```python
from build123d import *

# Parameters (mm, degrees)
SKICA1_R                = 2
P_IDAT_VYSUNUT_M3_DEPTH = 2


with BuildPart() as part:
    # Skica1 → Přidat vysunutím3 (new body)
    # profile 1 of 2: a face of its own
    with BuildSketch(Plane(origin=(0, 0, 0), x_dir=(1, 0, 0), z_dir=(0, 1, 0))):
        with BuildLine():
            Line((108.040914438, 105.971068272), (106.006427981, 34.226677149))
            ThreePointArc((106.006427981, 34.226677149), (110.004588085, 37.999997369), (113.994081517, 34.217515135))
            Line((113.994081517, 34.217515135), (112.040914438, 106))
            Line((112.040914438, 106), (110, 111.642221926))
            Line((110, 111.642221926), (108.040914438, 105.971068272))
        make_face()
    # profile 2 of 2: a face of its own
    with BuildSketch(Plane(origin=(0, 0, 0), x_dir=(1, 0, 0), z_dir=(0, 1, 0))):
        with BuildLine():
            ThreePointArc((106, 34), (107.171572875, 31.171572875), (110, 30))
            ThreePointArc((110, 30), (112.828427125, 31.171572875), (114, 34))
            Line((114, 34), (113.994081517, 34.217515135))
            ThreePointArc((113.994081517, 34.217515135), (110.004588085, 37.999997369), (106.006427981, 34.226677149))
            Line((106.006427981, 34.226677149), (106, 34))
        make_face()
        with Locations(Location((110, 34, 0), (0, 0, 270))):
            Circle(SKICA1_R, mode=Mode.SUBTRACT)
    extrude(amount=P_IDAT_VYSUNUT_M3_DEPTH)


solid = part.part
```
Here's how the part is built. I have some questions about the finished solid (model axes, mm). Coordinates: 2 decimals unless noted, no trailing zeros. Loops run counter-clockwise (first coordinate to the right, second up) from the corner with the lowest first, then second, coordinate; pieces in that order, holes last. Notation, with made-up numbers: (26, 82) - (67, 82) arc R15 cw to (67, 109) - close; hole circle Ø1 at (-1, 17). An arc over 180 degrees is marked (long way). Answer as CSV lines item,"result".
Q1. If we section it at A-A, the plane y = 0.35: Write out the boundary of the cut face in (x, z).
Response:
outline,"(106, -34) - (108.04, -105.97) - (110, -111.64) - (112.04, -106) - (114, -34) arc R4 ccw to start; hole circle Ø4 at (110, -34)"
Q2. If we section it at B-B, the plane x = 110.75: Write out the boundary of the cut face in (y, z), and give its area (3 significant figures).
Response:
outline,"(0, -109.57) - (2, -109.57) - (2, -35.85) - (0, -35.85) - close; (0, -32.15) - (2, -32.15) - (2, -30.07) - (0, -30.07) - close"
area,"152 mm2"
Q3. If we section it at C-C, the plane z = -93: Write out the boundary of the cut face in (x, y).
Response:
outline,"(107.67, 0) - (112.39, 0) - (112.39, 2) - (107.67, 2) - close"
Q4. If I drill on L1, parallel to X at y = 0.5, z = -34; L2, parallel to X at y = 0.65, z = -80.5; L3, parallel to X at y = 0.7, z = -45, over which ranges is the centre line in solid material (lowest first)? Write a range as [from, to].
Response:
L1,"[106, 108], [112, 114]"
L2,"[107.32, 112.73]"
L3,"[106.31, 113.7]"
Q5. If we section it at D-D, the plane x = 107.25: Write out the boundary of the cut face in (y, z), and give its area (3 significant figures).
Response:
outline,"(0, -78.08) - (2, -78.08) - (2, -31.1) - (0, -31.1) - close"
area,"94.0 mm2"
Q6. We'd pull the mould along X, two halves only. Please class faces 1 (the face through (110, 0, -62)), 2 (the face through (111.686, 0.986, -32.925)), 3 (the face through (111.035, 0.986, -108.782)): pulls with the +X half, pulls with the -X half, needs draft (parallel to the pull), parting line crosses it, or undercut.
Response:
face 1,"needs draft"
face 2,"undercut"
face 3,"pulls with the +X half"
